The model under review builds one solid part; all positions refer to its coordinate system, in mm. A direction names the side the tool comes from. Give positions to 0.01 mm unless a question says otherwise; leave off trailing zeros. Order: outer loops, then holes, each group sorted by start corner. A loop starts at its lowest first (then second) coordinate and runs counter-clockwise, first axis right, second up. Notation, with made-up numbers: (36, 70) -> (50, 70) arc R5 ccw to (50, 75) -> close; hole circle Ø7 at (-0.75, -37.75). An arc over 180 degrees is marked (long way). Answer as a JSON object with one key per item and string values. Group by question number.
from build123d import *

# Parameters (mm, degrees)
SKETCH1_W           = 100
SKETCH1_H           = 150
BOSS_EXTRUDE1_DEPTH = 4
SKETCH2_W           = 27
SKETCH2_H           = 19
CUT_EXTRUDE1_DEPTH  = 4
SKETCH2_4_W         = 12
SKETCH2_4_H         = 4
CUT_EXTRUDE2_DEPTH  = 4
SKETCH3_R           = 2.5
CUT_EXTRUDE3_DEPTH  = 4
SKETCH4_R           = 3
CUT_EXTRUDE4_DEPTH  = 4
FILLET1_R           = 2


with BuildPart() as part:
    # Sketch1 → Boss-Extrude1 (new body)
    with BuildSketch(Plane(origin=(0, 0, 0), x_dir=(1, 0, 0), z_dir=(0, 1, 0))):
        with Locations((50, 75)):
            Rectangle(SKETCH1_W, SKETCH1_H)
    extrude(amount=BOSS_EXTRUDE1_DEPTH)

    # Sketch2 → Cut-Extrude1 (cut)
    with BuildSketch(Plane(origin=(0, 4, 0), x_dir=(1, 0, 0), z_dir=(0, 1, 0))):
        with Locations((50, 107.008398101)):
            Rectangle(SKETCH2_W, SKETCH2_H)
    extrude(amount=-CUT_EXTRUDE1_DEPTH, mode=Mode.SUBTRACT)

    # Sketch2_4 → Cut-Extrude2 (cut)
    with BuildSketch(Plane(origin=(0, 4, 0), x_dir=(1, 0, 0), z_dir=(0, 1, 0))):
        with Locations((50, 95.508398101)):
            Rectangle(SKETCH2_4_W, SKETCH2_4_H)
    extrude(amount=-CUT_EXTRUDE2_DEPTH, mode=Mode.SUBTRACT)

    # Sketch3 → Cut-Extrude3 (cut)
    with BuildSketch(Plane(origin=(0, 4, 0), x_dir=(1, 0, 0), z_dir=(0, 1, 0))):
        with Locations((48.975949338, 73.129510144)):
            Circle(SKETCH3_R)
        with Locations((48.975949338, 54.212155816)):
            Circle(SKETCH3_R)
        with Locations((57.774718793, 64.110771453)):
            Circle(SKETCH3_R)
        with Locations((39.737241411, 64.110771453)):
            Circle(SKETCH3_R)
    extrude(amount=-CUT_EXTRUDE3_DEPTH, mode=Mode.SUBTRACT)

    # Sketch4 → Cut-Extrude4 (cut)
    with BuildSketch(Plane(origin=(0, 4, 0), x_dir=(1, 0, 0), z_dir=(0, 1, 0))):
        with Locations((56.881630687, 130.696209526)):
            Circle(SKETCH4_R)
        with Locations((41.869015261, 130.696209526)):
            Circle(SKETCH4_R)
    extrude(amount=-CUT_EXTRUDE4_DEPTH, mode=Mode.SUBTRACT)

    # Fillet1
    fillet1_edges = [part.edges().sort_by_distance(p)[0] for p in [
        (50, 4, 0),
        (0, 4, -75),
        (50, 4, -150),
        (0, 2, -150),
        (0, 2, 0),
        (100, 2, 0),
        (100, 2, -150),
        (100, 4, -75),
    ]]
    fillet(fillet1_edges, radius=FILLET1_R)


solid = part.part
1. Machinability: for faces 3 (the flat face through (49, 4, -76)), 4 (the flat face through (60, 2, -97.508)), which of the approach directions +Z, -Z, +X, -X, +Y, -Y give a long, thin tool a straight path to every point of the face, cutting with its end or side? Answer none if there is none.
2. Take a section at A-A on y = 3.3. Give the boundary of the cut face in (x, z).
3. Draft analysis for pull direction X (two halves, no side actions). For faces 1 (the flat face through (49, 0, -76)), 2 (the flat face through (56, 2, -95)), state which applies: pulls with the +X half, pulls with the -X half, needs draft (parallel to the pull), parting line crosses it, or undercut.
4. For pin 1 (3.5 mm diameter, centred on x = 56.88, z = -130.7, fed in from -Y); pin 2 (1.2 mm diameter, centred on x = 41.5, y = 3, fed in from -Z), all flat-tipped, find the tip position at first contact; note any pin that passes through.
5. For probe 1 along X at (y, z) = (0.3, -54.5); probe 2 along Z at (x, y) = (47, 1.6); probe 3 along Z at (x, y) = (61, 3.3), list the stretches that pass through material, from the lowest coordinate up. Write a range as [from, to].
Checks:
{
 "1": {"face 3": "+Z, -Z, +X, -X, +Y", "face 4": "+Y, -Y"},
 "2": {"outline": "(0.48, -148) arc R1.52 ccw to (2, -149.52) -> (98, -149.52) arc R1.52 ccw to (99.52, -148) -> (99.52, -2) arc R1.52 ccw to (98, -0.48) -> (2, -0.48) arc R1.52 ccw to (0.48, -2) -> close; hole (36.5, -116.51) -> (63.5, -116.51) -> (63.5, -97.51) -> (56, -97.51) -> (56, -93.51) -> (44, -93.51) -> (44, -97.51) -> (36.5, -97.51) -> close; hole circle Ø5 at (39.74, -64.11); hole circle Ø6 at (41.87, -130.7); hole circle Ø5 at (48.98, -73.13); hole circle Ø5 at (48.98, -54.21); hole circle Ø6 at (56.88, -130.7); hole circle Ø5 at (57.77, -64.11)"},
 "3": {"face 1": "needs draft", "face 2": "undercut"},
 "4": {"pin 1": "passes through", "pin 2": "stops at z = -149.96"},
 "5": {"probe 1": "x = [0, 46.49], [51.46, 100]", "probe 2": "z = [-150, -116.51], [-93.51, -74.66], [-71.6, -55.74], [-52.68, 0]", "probe 3": "z = [-149.52, -116.51], [-97.51, -0.48]"}
}
